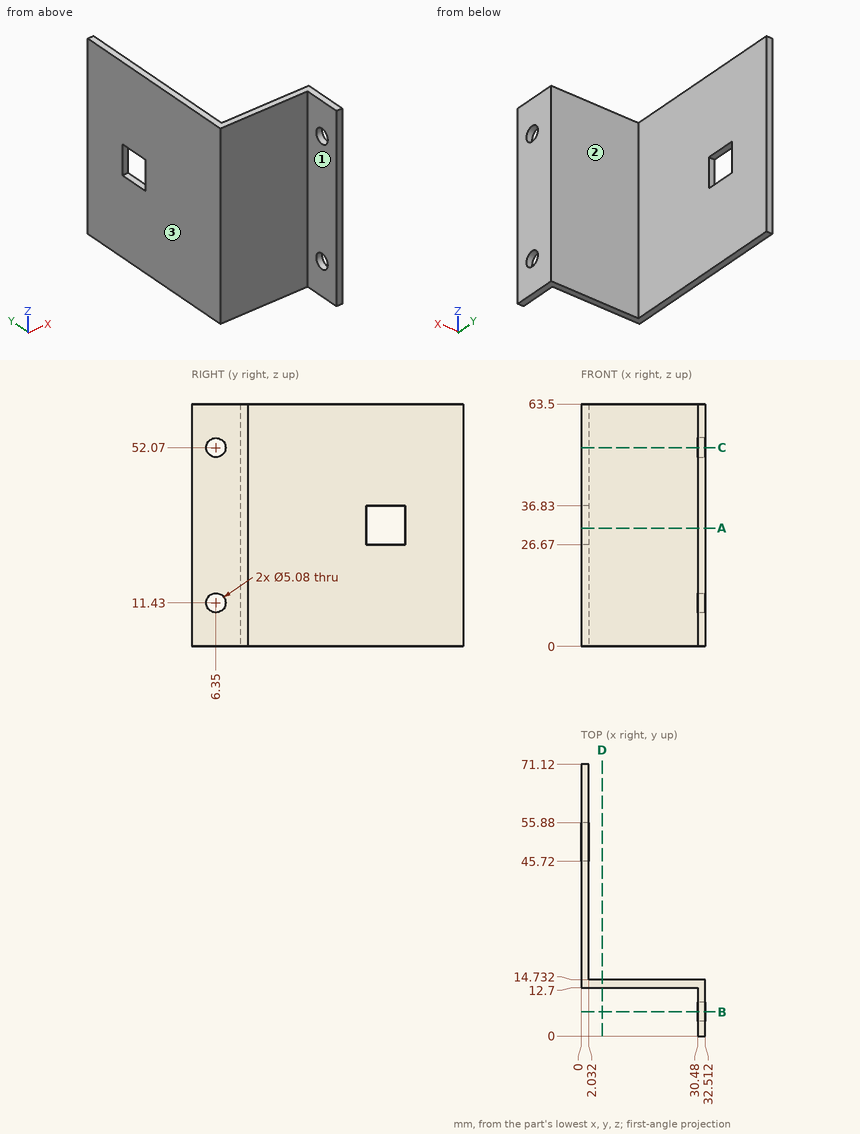
Geometry: see drawing. Coordinates: mm, zero at the bounding-box minimum. A direction names the side the tool comes from. Give positions to 0.01 mm unless a question says otherwise; leave off trailing zeros. Loops run counter-clockwise (first coordinate to the right, second up) from the corner with the lowest first, then second, coordinate; pieces in that order, holes last. Notation, with made-up numbers: (40, 7.5) - (58, 7.5) arc R27 ccw to (58, 31.5) - close; hole circle Ø4 at (-23, 1.25). An arc over 180 degrees is marked (long way). Answer as CSV lines item,"result". Start each with the question number.
1. Section D-D, the plane x = 5.5. Return loops of the section in (y, z).
2. Pin query (flat end, axial travel): P1, Ø1, axis at x = 0.5, z = 33, coming from the -Y side; P2, Ø9, axis at x = 14.5, z = 16, coming from the +Y side; P3, Ø6, axis at y = 6.35, z = 52.07, coming from the -X side. Return the tip coordinate at first contact, or that it passes through.
3. Reachability of the marked faces 1, 2 and 3 from +Z, -Z, +X, -X, +Y, -Y: full face, straight path, thin tool, end or side. Return the list, or none.
4. Ray query, L1, parallel to Y at x = 32, z = 52; L2, parallel to Y at x = 13.5, z = 54; L3, parallel to Z at x = 31, y = 6. Return the intervals inside material, ascending.
5. Section A-A, the plane z = 31. Return loops of the section in (x, y), plus the area to 3 significant figures.
6. Section B-B, the plane y = 6.35. Return loops of the section in (x, z).
7. Section C-C, the plane z = 52.07. Return loops of the section in (x, y).
Answers:
1,outline,"(12.7, 0) - (14.73, 0) - (14.73, 63.5) - (12.7, 63.5) - close"
2,P1,"stops at y = 12.7"
2,P2,"stops at y = 14.73"
2,P3,"stops at x = 30.48"
3,face 1,"+Z, -Z, -X, -Y"
3,face 2,"+Z, -Z, +X, +Y"
3,face 3,"+Z, -Z, -X, +Y, -Y"
4,L1,"y = 0 to 3.81, 8.89 to 14.73"
4,L2,"y = 12.7 to 14.73"
4,L3,"z = 0 to 8.91, 13.95 to 49.55, 54.59 to 63.5"
5,outline,"(0, 12.7) - (30.48, 12.7) - (30.48, 0) - (32.51, 0) - (32.51, 14.73) - (2.03, 14.73) - (2.03, 45.72) - (0, 45.72) - close; (0, 55.88) - (2.03, 55.88) - (2.03, 71.12) - (0, 71.12) - close"
5,area,"186 mm2"
6,outline,"(30.48, 0) - (32.51, 0) - (32.51, 8.89) - (30.48, 8.89) - close; (30.48, 13.97) - (32.51, 13.97) - (32.51, 49.53) - (30.48, 49.53) - close; (30.48, 54.61) - (32.51, 54.61) - (32.51, 63.5) - (30.48, 63.5) - close"
7,outline,"(0, 12.7) - (30.48, 12.7) - (30.48, 8.89) - (32.51, 8.89) - (32.51, 14.73) - (2.03, 14.73) - (2.03, 71.12) - (0, 71.12) - close; (30.48, 0) - (32.51, 0) - (32.51, 3.81) - (30.48, 3.81) - close"
